```python
from build123d import *

# Parameters (mm, degrees)
SKETCH_1_W                                      = 64
SKETCH_1_H                                      = 8
SERVO_FOOT_DEPTH                                = 24
SKETCH_2_W                                      = 64
SKETCH_2_H                                      = 71
SERVO_FACE_PLATE_DEPTH                          = 6
MG995_BODY_WINDOW_REFERENCE_DEPTH               = 87.406018309
MG995_BODY_WINDOW_REFERENCE_DEPTH_BACK          = 87.406018309
SKETCH_3_W                                      = 41.7
SKETCH_3_H                                      = 21
MG995_47P2X10_REFERENCE_SLOTS_VERIFY_DEPTH      = 87.406018309
MG995_47P2X10_REFERENCE_SLOTS_VERIFY_DEPTH_BACK = 87.406018309
SKETCH_4_W                                      = 4
SKETCH_4_H                                      = 5
SERVO_FOOT_M3_DEPTH                             = 87.406018309
SERVO_FOOT_M3_DEPTH_BACK                        = 87.406018309
SKETCH_5_R                                      = 1.7


with BuildPart() as part:
    # 草图1 → Servo_foot (new body)
    with BuildSketch(Plane.XY):
        with Locations((11, 4)):
            Rectangle(SKETCH_1_W, SKETCH_1_H)
    extrude(amount=SERVO_FOOT_DEPTH)

    # 草图2 → Servo_face_plate (add)
    with BuildSketch(Plane.XY):
        with Locations((11, 35.5)):
            Rectangle(SKETCH_2_W, SKETCH_2_H)
    extrude(amount=SERVO_FACE_PLATE_DEPTH)

    # 草图3 → MG995_body_window_REFERENCE (cut, two sides: drawn at the far end of the back side and taken through both)
    with BuildSketch(Plane.XY.offset(-MG995_BODY_WINDOW_REFERENCE_DEPTH_BACK)):
        with Locations((10.35, 60)):
            Rectangle(SKETCH_3_W, SKETCH_3_H)
    extrude(amount=MG995_BODY_WINDOW_REFERENCE_DEPTH + MG995_BODY_WINDOW_REFERENCE_DEPTH_BACK, mode=Mode.SUBTRACT)

    # 草图4 → MG995_47p2x10_reference_slots_VERIFY (cut, two sides: drawn at the far end of the back side and taken through both)
    with BuildSketch(Plane.XY.offset(-MG995_47P2X10_REFERENCE_SLOTS_VERIFY_DEPTH_BACK)):
        with Locations((-13.6, 55)):
            Rectangle(SKETCH_4_W, SKETCH_4_H)
        with Locations((-13.6, 65)):
            Rectangle(SKETCH_4_W, SKETCH_4_H)
        with Locations((33.6, 55)):
            Rectangle(SKETCH_4_W, SKETCH_4_H)
        with Locations((33.6, 65)):
            Rectangle(SKETCH_4_W, SKETCH_4_H)
    extrude(amount=MG995_47P2X10_REFERENCE_SLOTS_VERIFY_DEPTH + MG995_47P2X10_REFERENCE_SLOTS_VERIFY_DEPTH_BACK, mode=Mode.SUBTRACT)

    # 草图5 → Servo_foot_M3 (cut, two sides: drawn at the far end of the back side and taken through both)
    with BuildSketch(Plane(origin=(0, 0, 0), x_dir=(1, 0, 0), z_dir=(0, 1, 0)).offset(-SERVO_FOOT_M3_DEPTH_BACK)):
        with Locations(Location((-9, -3, 0), (0, 0, 270))):
            Circle(SKETCH_5_R)
        with Locations(Location((-9, -21, 0), (0, 0, 270))):
            Circle(SKETCH_5_R)
        with Locations(Location((31, -3, 0), (0, 0, 270))):
            Circle(SKETCH_5_R)
        with Locations(Location((31, -21, 0), (0, 0, 270))):
            Circle(SKETCH_5_R)
    extrude(amount=SERVO_FOOT_M3_DEPTH + SERVO_FOOT_M3_DEPTH_BACK, mode=Mode.SUBTRACT)


solid = part.part
```
Read the model definition and answer for the solid it produces. Units are mm, in the model's axes. A direction names the side the tool comes from. Give positions to 0.01 mm unless a question says otherwise; leave off trailing zeros. Write each loop counter-clockwise with the first axis right and the second up, starting at its lowest first coordinate (ties: lowest second). Pieces come first, ordered by that corner, then holes. Notation, with made-up numbers: M -15.75,4.5 L 29.25,4.5 A12 ccw 29.25,23.5 Z; hole C -12,11 d1. An arc over 180 degrees is marked long. Put each result on its own line as item: value. Start each with the question number.
1. The part is cut by section A-A, the plane z = 3. Give the number of separate pieces and of enclosed holes in the cut face, and give its area (3 significant figures).
2. The part is cut by section B-B, the plane x = 22. Give the vertices of the cut face in (y, z), and give its area (3 significant figures).
3. Each of these flat-tipped pins is pushed along its axis until it touches: pin 1 Ø2 at (x, z) = (-9, 3) entering from +Y; pin 2 Ø5.5 at (x, z) = (31, 21) entering from +Y; pin 3 Ø19 at (x, y) = (5, 32.5) entering from +Z. Where does it stop, or does it pass through?
4. Consider line 1 along Z through (x, y) = (-9, 5); line 2 along X through (y, z) = (2.5, 21); line 3 along X through (y, z) = (51, 3). Determine where each line is inside the solid, lowest interval first.
5. For a pull along Y with two mould halves and no side action, classify faces 3 (the flat face through (-11.6, 55, 3)), 4 (the flat face through (43, 27.4, 5.7)), 5 (the flat face through (11, 0, 12)) as released by +Y, released by -Y, zero draft, split by the parting line, or undercut.
6. Which of the six approach directions +Z, -Z, +X, -X, +Y, -Y give full straight-line access (tool end or side, diameter ignored) to faces 1 (the flat face through (-10.5, 60, 5)), 2 (the cylindrical face through (-9.65, 3.94, 22.57))?
7. The part is cut by section D-D, the plane z = 21. Give the vertices of the cut face in (x, y).
8. The part is cut by section C-C, the plane y = 66. Give the vertices of the cut face in (x, z).
Final values:
1. separate pieces: 4
1. enclosed holes: 2
1. area: 3,220 mm²
2. outline: M 0,0 L 49.5,0 L 49.5,6 L 8,6 L 8,24 L 0,24 Z; M 70.5,0 L 71,0 L 71,6 L 70.5,6 Z
2. area: 444 mm²
3. pin 1: passes through
3. pin 2: stops at y = 8
3. pin 3: stops at z = 6
4. line 1: z = 0 to 1.3, 4.7 to 19.3, 22.7 to 24
4. line 2: x = -21 to -10.7, -7.3 to 29.3, 32.7 to 43
4. line 3: x = -21 to -10.7, 32.7 to 43
5. face 3: undercut
5. face 4: zero draft
5. face 5: released by -Y
6. face 1: +Z, -Z
6. face 2: +Y, -Y
7. outline: M -21,0 L -10.7,0 L -10.7,8 L -21,8 Z; M -7.3,0 L 29.3,0 L 29.3,8 L -7.3,8 Z; M 32.7,0 L 43,0 L 43,8 L 32.7,8 Z
8. outline: M -21,0 L -15.6,0 L -15.6,6 L -21,6 Z; M -11.6,0 L -10.5,0 L -10.5,2.2 A1.7 cw -10.5,3.8 L -10.5,6 L -11.6,6 Z; M 31.2,0 L 31.6,0 L 31.6,1.41 A1.7 cw 31.2,1.31 Z; M 31.2,4.69 A1.7 cw 31.6,4.59 L 31.6,6 L 31.2,6 Z; M 35.6,0 L 43,0 L 43,6 L 35.6,6 Z
